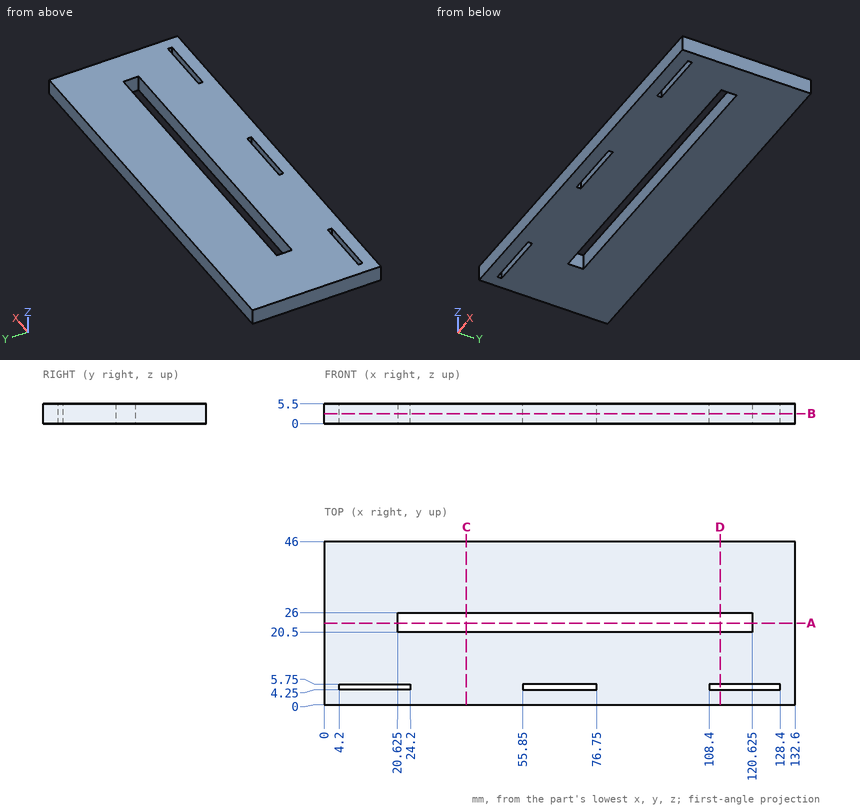
Job drawing, mm, ordinate dimensions from the low corner. One solid piece. Give positions to 0.01 mm unless a question says otherwise; leave off trailing zeros. Order: outer loops, then holes, each group sorted by start corner. A loop starts at its lowest first (then second) coordinate and runs counter-clockwise, first axis right, second up. Notation, with made-up numbers: (84, -16.5) - (126, -16.5) arc R23 cw to (126, -7.5) - close; hole circle Ø2 at (17.5, -18.5). An arc over 180 degrees is marked (long way). Return JSON: item names as keys, results as strings.
1) Cut at A-A, the plane y = 23. Give the cut face in (x, z) (1 decimal).
Geometry says:
{"outline": "(0, 0) - (20.6, 0) - (20.6, 5.5) - (0, 5.5) - close; (120.6, 0) - (132.6, 0) - (132.6, 5.5) - (120.6, 5.5) - close"}
2) Cut at C-C, the plane x = 40. Give the cut face in (y, z), plus the area to 3 significant figures.
Geometry says:
{"outline": "(0, 0) - (20.5, 0) - (20.5, 5.5) - (0, 5.5) - close; (26, 0) - (46, 0) - (46, 5.5) - (26, 5.5) - close", "area": "223 mm²"}
3) Cut at D-D, the plane x = 111.5. Give the cut face in (y, z).
Geometry says:
{"outline": "(0, 0) - (4.25, 0) - (4.25, 5.5) - (0, 5.5) - close; (5.75, 0) - (20.5, 0) - (20.5, 5.5) - (5.75, 5.5) - close; (26, 0) - (46, 0) - (46, 5.5) - (26, 5.5) - close"}
4) Probe line 1 (X direction, y = 5, z = 4.4); line 2 (Y direction, x = 57, z = 3.7); line 3 (Y direction, x = 11, z = 3.25). List the from-to ranges inside material, lowest first. Write a range as from..to.
Geometry says:
{"line 1": "0..4.2, 24.2..55.85, 76.75..108.4, 128.4..132.6", "line 2": "0..4.25, 5.75..20.5, 26..46", "line 3": "0..4.25, 5.75..46"}
5) Cut at B-B, the plane z = 2.8. Count the separate pieces of the cut face and the enclosed holes in it, plus the area to 3 significant figures.
Geometry says:
{"separate pieces": "1", "enclosed holes": "4", "area": "5,460 mm²"}
6) Flat gauge pin, fed straight in: P1, Ø3, axis at x = 25.5, z = 1.5, coming from the -Y side. Where does the tip first touch, or does it go through?
Geometry says:
{"P1": "y = 0"}
